Input: dimensioned drawing with shaded views. Units: mm. Origin: part minimum x, y, z. A direction names the side the tool comes from. Round coordinates to 2 decimals unless told otherwise and drop trailing zeros. Order: outer loops, then holes, each group sorted by start corner. A loop starts at its lowest first (then second) coordinate and runs counter-clockwise, first axis right, second up. Notation, with made-up numbers: M 22.25,71.5 L 78.25,71.5 A14 ccw 78.25,95.5 Z; hole C 76,11 d8. An arc over 180 degrees is marked long. Use one line per item in the form item = value. Start each with the question number.
Q1. Section D-D (x = 11.5). Return the cut outline in (y, z).
Q2. Section C-C (z = 24). Return the cut outline in (x, y), plus the area to 3 significant figures.
Q3. Section A-A (x = 24). Return the cut outline in (y, z), plus the area to 3 significant figures.
Q4. Reachability of the marked faces 1 and 2 from +Z, -Z, +X, -X, +Y, -Y: full face, straight path, thin tool, end or side. Return the list, or none.
Q5. Material intervals for probe 1 along Z at (x, y) = (4.5, 2.25); probe 2 along X at (y, z) = (2, 15); probe 3 along Z at (x, y) = (7, 1.5), sorted ascending.
Q6. Contact query for flat-ended pins moving along their axis: pin 1 (2 mm diameter, centred on x = 5.597, z = 34.625, fed in from -Y); pin 2 (2 mm diameter, centred on x = 19.5, y = 3, fed in from +Z); pin 3 (6 mm diameter, centred on x = 24, z = 2.75, fed in from +Y); pin 4 (3 mm diameter, centred on x = 41, y = 1.5, fed in from +Z). Output: stop coordinate, or through.
Q7. Section B-B (z = 45.25). Return the cut outline in (x, y).
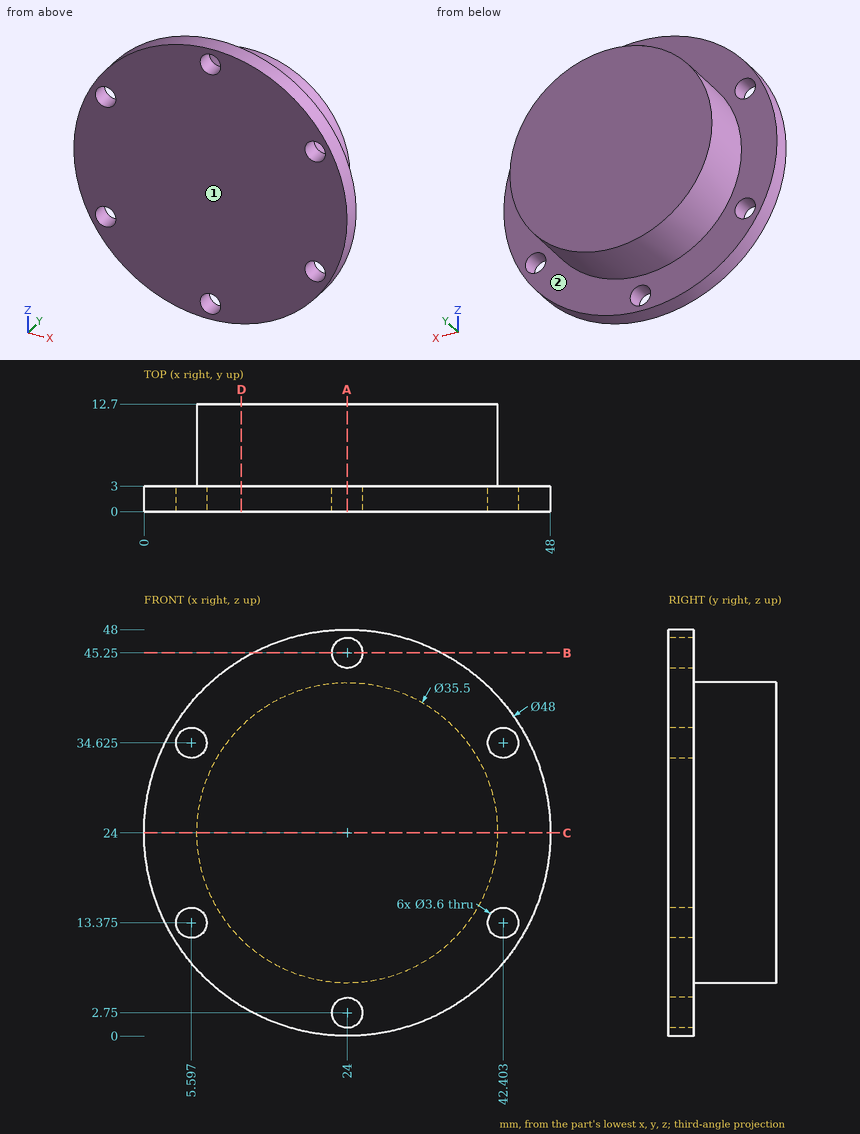
Results list:
q1.outline = M 0,3.51 L 3,3.51 L 3,11.4 L 12.7,11.4 L 12.7,36.6 L 3,36.6 L 3,44.49 L 0,44.49 Z
q2.outline = M 0,0 L 48,0 L 48,3 L 41.75,3 L 41.75,12.7 L 6.25,12.7 L 6.25,3 L 0,3 Z
q2.area = 488 mm2
q3.outline = M 0,0 L 3,0 L 3,0.95 L 0,0.95 Z; M 0,4.55 L 3,4.55 L 3,6.25 L 12.7,6.25 L 12.7,41.75 L 3,41.75 L 3,43.45 L 0,43.45 Z; M 0,47.05 L 3,47.05 L 3,48 L 0,48 Z
q3.area = 467 mm2
q4.face_1 = +Z, -Z, +X, -X, -Y
q4.face_2 = +Y
q5.probe_1 = 10.01 to 11.95, 14.8 to 33.2, 36.05 to 37.99
q5.probe_2 = 1.75 to 4.82, 6.37 to 41.63, 43.18 to 46.25
q5.probe_3 = 7.06 to 12.25, 14.5 to 33.5, 35.75 to 40.94
q6.pin_1 = through
q6.pin_2 = 47.74
q6.pin_3 = 3
q6.pin_4 = 42.32
q7.outline = M 12.84,0 L 22.2,0 L 22.2,3 L 12.84,3 Z; M 25.8,0 L 35.16,0 L 35.16,3 L 25.8,3 Z
